Geometry check sheet. Reference: the model listing, model coordinates, mm. A direction names the side the tool comes from. Round coordinates to 2 decimals unless told otherwise and drop trailing zeros. Write each loop counter-clockwise with the first axis right and the second up, starting at its lowest first coordinate (ties: lowest second). Pieces come first, ordered by that corner, then holes. Notation, with made-up numbers: (21, 1) -> (48, 1) arc R21 ccw to (48, 35) -> close; hole circle Ø7 at (-22, 14.5). An arc over 180 degrees is marked (long way). Return JSON: item names as keys, results as strings. Group by question number.
from build123d import *

# Parameters (mm, degrees)
F0_R     = 5.5
F1_DEPTH = 15
F2_R     = 11.5
F3_DEPTH = 5
F5_D     = 3.5


with BuildPart() as f1:
    # F0 (on Top) → F1 (new body)
    with BuildSketch(Plane.XY):
        with BuildLine():
            ThreePointArc((-18, 4), (-14, 0), (-18, -4))
            Line((-18, -4), (-30, -4))
            Line((-30, -4), (-30, -6))
            Line((-30, -6), (-3.83581, -14.501261))
            ThreePointArc((-3.83581, -14.501261), (15, 0), (-3.83581, 14.501261))
            Line((-3.83581, 14.501261), (-30, 6))
            Line((-30, 6), (-30, 4))
            Line((-30, 4), (-18, 4))
        make_face()
        Circle(F0_R, mode=Mode.SUBTRACT)
    extrude(amount=F1_DEPTH)

    # F2 (on face) → F3 (cut)
    with BuildSketch(Plane.XY.offset(15)):
        Circle(F2_R)
    extrude(amount=-F3_DEPTH, mode=Mode.SUBTRACT)

    # F5 (through all)
    with Locations(Plane.XY.offset(10)):
        with Locations((0, 8), (8, 0), (0, -8), (-8, 0)):
            Hole(F5_D / 2)


solid = f1.part
1) Material ranges on probe 1 along Y at (x, z) = (0, 4); probe 2 along X at (y, z) = (3.5, 2); probe 3 along Y at (x, z) = (8, 4.25), recorded low to high. Write a range as [from, to].
2) Sectioned sample at C-C on y = 0. Enter the section's corners in (x, z).
3) Sectioned sample at D-D on z = 5. Enter the section's corners in (x, y).
4) Go/stop test with flat-tipped pins: P1, Ø1, axis at y = 3, z = 2.5, coming from the +X side; P2, Ø2, axis at x = -6.5, z = 4, coming from the +Y side; P3, Ø14, axis at x = 0, y = 0, coming from the -Z side; P4, Ø12.5, axis at x = 0, y = 0, coming from the +Z side. Record where each tip stops, or that it passes through.
5) Sectioned sample at A-A on x = 0. Enter the section's corners in (y, z), and give its area (3 significant figures).
6) Sectioned sample at B-B on z = 11.5. Enter the section's corners in (x, y).
7) Tool access check on faces 5 (the face through (-24, 4, 7)), 6 (the face through (15, 0, 7)). Record the directions out of +Z, -Z, +X, -X, +Y, -Y that give a thin tool (end or side, any length) a straight path to the whole face; none if there is none.
8) Mould release check, pull along X, two halves, no side actions. Record for faces 1 (the face through (5, 3, 10)), 2 (the face through (-17.1, -10.19, 7.4)), 3 (the face through (-24, -4, 7)), 4 (the face through (-1.5, 11.4, 12.5)): +X half, -X half, draft (parallel to the pull), parting line (faces both ways), or undercut.
Evaluation:
{
 "1": {"probe 1": "y = [-15, -9.75], [-6.25, -5.5], [5.5, 6.25], [9.75, 15]", "probe 2": "x = [-16.06, -4.24], [4.24, 14.59]", "probe 3": "y = [-12.69, -1.75], [1.75, 12.69]"},
 "2": {"outline": "(-14, 0) -> (-9.75, 0) -> (-9.75, 10) -> (-11.5, 10) -> (-11.5, 15) -> (-14, 15) -> close; (-6.25, 0) -> (-5.5, 0) -> (-5.5, 10) -> (-6.25, 10) -> close; (5.5, 0) -> (6.25, 0) -> (6.25, 10) -> (5.5, 10) -> close; (9.75, 0) -> (15, 0) -> (15, 15) -> (11.5, 15) -> (11.5, 10) -> (9.75, 10) -> close"},
 "3": {"outline": "(-30, -6) -> (-3.84, -14.5) arc R15 ccw (long way) to (-3.84, 14.5) -> (-30, 6) -> (-30, 4) -> (-18, 4) arc R4 cw to (-18, -4) -> (-30, -4) -> close; hole circle Ø3.5 at (-8, 0); hole circle Ø11 at (0, 0); hole circle Ø3.5 at (0, -8); hole circle Ø3.5 at (0, 8); hole circle Ø3.5 at (8, 0)"},
 "4": {"P1": "stops at x = 14.79", "P2": "stops at y = 13.96", "P3": "stops at z = 0", "P4": "stops at z = 10"},
 "5": {"outline": "(-15, 0) -> (-9.75, 0) -> (-9.75, 10) -> (-11.5, 10) -> (-11.5, 15) -> (-15, 15) -> close; (-6.25, 0) -> (-5.5, 0) -> (-5.5, 10) -> (-6.25, 10) -> close; (5.5, 0) -> (6.25, 0) -> (6.25, 10) -> (5.5, 10) -> close; (9.75, 0) -> (15, 0) -> (15, 15) -> (11.5, 15) -> (11.5, 10) -> (9.75, 10) -> close", "area": "155 mm2"},
 "6": {"outline": "(-30, -6) -> (-3.84, -14.5) arc R15 ccw (long way) to (-3.84, 14.5) -> (-30, 6) -> (-30, 4) -> (-18, 4) arc R4 cw to (-18, -4) -> (-30, -4) -> close; hole circle Ø23 at (0, 0)"},
 "7": {"face 5": "+Z, -Z, -X", "face 6": "+Z, -Z"},
 "8": {"face 1": "undercut", "face 2": "-X half", "face 3": "draft", "face 4": "undercut"}
}
